Build history of the part. All positions in model axes, mm. A direction names the side the tool comes from. Round coordinates to 2 decimals unless told otherwise and drop trailing zeros. Loops run counter-clockwise (first coordinate to the right, second up) from the corner with the lowest first, then second, coordinate; pieces in that order, holes last.
from build123d import *

# Parameters (mm, degrees)
CROQUIS1_R              = 44.1
CROQUIS1_R_2            = 15.875
SALIENTE_EXTRUIR1_DEPTH = 15.875
SALIENTE_EXTRUIR2_DEPTH = 15.875
MATRIZC1_DEPTH          = 15.875


# Read off the part's stored shape, not the designer's step: MatrizC1
with BuildPart() as part:
    # Croquis1 → Saliente-Extruir1 (new body)
    with BuildSketch(Plane.XY):
        Circle(CROQUIS1_R)
        Circle(CROQUIS1_R_2, mode=Mode.SUBTRACT)
    extrude(amount=SALIENTE_EXTRUIR1_DEPTH)

    # Croquis2 → Saliente-Extruir2 (add)
    with BuildSketch(Plane.XY.offset(15.875)):
        Polygon((-1, 50.6), (1, 50.6), (2.815859205, 42.731276779), (-2.815859205, 42.731276779), align=None)
    extrude(amount=-SALIENTE_EXTRUIR2_DEPTH)

    # MatrizC1 outline → MatrizC1 (add)
    with BuildSketch(Plane.XY):
        with BuildLine():
            ThreePointArc((-13.826153616, 41.876574313), (-11.413919889, 42.59732894), (-8.964486889, 43.179253987))
            Line((-8.964486889, 43.179253987), (-12.130317856, 49.134665855))
            Line((-12.130317856, 49.134665855), (-14.062169508, 48.617027765))
            Line((-14.062169508, 48.617027765), (-13.826153616, 41.876574313))
        make_face()
        with BuildLine():
            ThreePointArc((8.964486889, 43.179253987), (11.413919889, 42.59732894), (13.826153616, 41.876574313))
            Line((13.826153616, 41.876574313), (14.062169508, 48.617027765))
            Line((14.062169508, 48.617027765), (12.130317856, 49.134665855))
            Line((12.130317856, 49.134665855), (8.964486889, 43.179253987))
        make_face()
        with BuildLine():
            ThreePointArc((19.83464269, 39.387776649), (22.05, 38.191720307), (24.193493831, 36.87119277))
            Line((24.193493831, 36.87119277), (26.166025404, 43.320885431))
            Line((26.166025404, 43.320885431), (24.433974596, 44.320885431))
            Line((24.433974596, 44.320885431), (19.83464269, 39.387776649))
        make_face()
        with BuildLine():
            ThreePointArc((29.353100371, 32.912087424), (31.18340905, 31.18340905), (32.912087424, 29.353100371))
            Line((32.912087424, 29.353100371), (36.486709909, 35.072496347))
            Line((36.486709909, 35.072496347), (35.072496347, 36.486709909))
            Line((35.072496347, 36.486709909), (29.353100371, 32.912087424))
        make_face()
        with BuildLine():
            ThreePointArc((36.87119277, 24.193493831), (38.191720307, 22.05), (39.387776649, 19.83464269))
            Line((39.387776649, 19.83464269), (44.320885431, 24.433974596))
            Line((44.320885431, 24.433974596), (43.320885431, 26.166025404))
            Line((43.320885431, 26.166025404), (36.87119277, 24.193493831))
        make_face()
        with BuildLine():
            ThreePointArc((41.876574313, 13.826153616), (42.597328939, 11.413919889), (43.179253986, 8.964486889))
            Line((43.179253986, 8.964486889), (49.134665855, 12.130317856))
            Line((49.134665855, 12.130317856), (48.617027765, 14.062169508))
            Line((48.617027765, 14.062169508), (41.876574313, 13.826153616))
        make_face()
        with BuildLine():
            ThreePointArc((44.028136522, 2.51658388), (44.1, 0), (44.028136522, -2.51658388))
            Line((44.028136522, -2.51658388), (50.6, -1))
            Line((50.6, -1), (50.6, 1))
            Line((50.6, 1), (44.028136522, 2.51658388))
        make_face()
        with BuildLine():
            ThreePointArc((43.179253986, -8.964486889), (42.597328939, -11.413919889), (41.876574313, -13.826153616))
            Line((41.876574313, -13.826153616), (48.617027765, -14.062169508))
            Line((48.617027765, -14.062169508), (49.134665855, -12.130317856))
            Line((49.134665855, -12.130317856), (43.179253986, -8.964486889))
        make_face()
        with BuildLine():
            ThreePointArc((39.387776649, -19.83464269), (38.191720307, -22.05), (36.871192769, -24.193493831))
            Line((36.871192769, -24.193493831), (43.320885431, -26.166025404))
            Line((43.320885431, -26.166025404), (44.320885431, -24.433974596))
            Line((44.320885431, -24.433974596), (39.387776649, -19.83464269))
        make_face()
        with BuildLine():
            ThreePointArc((32.912087424, -29.353100371), (31.18340905, -31.18340905), (29.353100371, -32.912087424))
            Line((29.353100371, -32.912087424), (35.072496347, -36.486709909))
            Line((35.072496347, -36.486709909), (36.486709909, -35.072496347))
            Line((36.486709909, -35.072496347), (32.912087424, -29.353100371))
        make_face()
        with BuildLine():
            ThreePointArc((24.193493831, -36.871192769), (22.05, -38.191720307), (19.83464269, -39.387776649))
            Line((19.83464269, -39.387776649), (24.433974596, -44.320885431))
            Line((24.433974596, -44.320885431), (26.166025404, -43.320885431))
            Line((26.166025404, -43.320885431), (24.193493831, -36.871192769))
        make_face()
        with BuildLine():
            ThreePointArc((13.826153616, -41.876574313), (11.413919889, -42.597328939), (8.964486889, -43.179253986))
            Line((8.964486889, -43.179253986), (12.130317856, -49.134665855))
            Line((12.130317856, -49.134665855), (14.062169508, -48.617027765))
            Line((14.062169508, -48.617027765), (13.826153616, -41.876574313))
        make_face()
        with BuildLine():
            ThreePointArc((2.51658388, -44.028136522), (0, -44.1), (-2.51658388, -44.028136522))
            Line((-2.51658388, -44.028136522), (-1, -50.6))
            Line((-1, -50.6), (1, -50.6))
            Line((1, -50.6), (2.51658388, -44.028136522))
        make_face()
        with BuildLine():
            ThreePointArc((-8.964486889, -43.179253986), (-11.413919889, -42.597328939), (-13.826153616, -41.876574313))
            Line((-13.826153616, -41.876574313), (-14.062169508, -48.617027765))
            Line((-14.062169508, -48.617027765), (-12.130317856, -49.134665855))
            Line((-12.130317856, -49.134665855), (-8.964486889, -43.179253986))
        make_face()
        with BuildLine():
            ThreePointArc((-19.83464269, -39.387776649), (-22.05, -38.191720307), (-24.193493831, -36.871192769))
            Line((-24.193493831, -36.871192769), (-26.166025404, -43.320885431))
            Line((-26.166025404, -43.320885431), (-24.433974596, -44.320885431))
            Line((-24.433974596, -44.320885431), (-19.83464269, -39.387776649))
        make_face()
        with BuildLine():
            ThreePointArc((-29.353100371, -32.912087424), (-31.18340905, -31.18340905), (-32.912087424, -29.353100371))
            Line((-32.912087424, -29.353100371), (-36.486709909, -35.072496347))
            Line((-36.486709909, -35.072496347), (-35.072496347, -36.486709909))
            Line((-35.072496347, -36.486709909), (-29.353100371, -32.912087424))
        make_face()
        with BuildLine():
            ThreePointArc((-36.871192769, -24.193493831), (-38.191720307, -22.05), (-39.387776649, -19.83464269))
            Line((-39.387776649, -19.83464269), (-44.320885431, -24.433974596))
            Line((-44.320885431, -24.433974596), (-43.320885431, -26.166025404))
            Line((-43.320885431, -26.166025404), (-36.871192769, -24.193493831))
        make_face()
        with BuildLine():
            ThreePointArc((-41.876574313, -13.826153616), (-42.597328939, -11.413919889), (-43.179253986, -8.964486889))
            Line((-43.179253986, -8.964486889), (-49.134665855, -12.130317856))
            Line((-49.134665855, -12.130317856), (-48.617027765, -14.062169508))
            Line((-48.617027765, -14.062169508), (-41.876574313, -13.826153616))
        make_face()
        with BuildLine():
            ThreePointArc((-44.028136522, -2.51658388), (-44.1, 0), (-44.028136522, 2.51658388))
            Line((-44.028136522, 2.51658388), (-50.6, 1))
            Line((-50.6, 1), (-50.6, -1))
            Line((-50.6, -1), (-44.028136522, -2.51658388))
        make_face()
        with BuildLine():
            ThreePointArc((-43.179253986, 8.964486889), (-42.597328939, 11.413919889), (-41.876574313, 13.826153616))
            Line((-41.876574313, 13.826153616), (-48.617027765, 14.062169508))
            Line((-48.617027765, 14.062169508), (-49.134665855, 12.130317856))
            Line((-49.134665855, 12.130317856), (-43.179253986, 8.964486889))
        make_face()
        with BuildLine():
            ThreePointArc((-39.387776649, 19.83464269), (-38.191720307, 22.05), (-36.87119277, 24.193493831))
            Line((-36.87119277, 24.193493831), (-43.320885431, 26.166025404))
            Line((-43.320885431, 26.166025404), (-44.320885431, 24.433974596))
            Line((-44.320885431, 24.433974596), (-39.387776649, 19.83464269))
        make_face()
        with BuildLine():
            ThreePointArc((-32.912087424, 29.353100371), (-31.18340905, 31.18340905), (-29.353100371, 32.912087424))
            Line((-29.353100371, 32.912087424), (-35.072496347, 36.486709909))
            Line((-35.072496347, 36.486709909), (-36.486709909, 35.072496347))
            Line((-36.486709909, 35.072496347), (-32.912087424, 29.353100371))
        make_face()
        with BuildLine():
            ThreePointArc((-24.193493831, 36.87119277), (-22.05, 38.191720307), (-19.83464269, 39.387776649))
            Line((-19.83464269, 39.387776649), (-24.433974596, 44.320885431))
            Line((-24.433974596, 44.320885431), (-26.166025404, 43.320885431))
            Line((-26.166025404, 43.320885431), (-24.193493831, 36.87119277))
        make_face()
    extrude(amount=MATRIZC1_DEPTH)


solid = part.part
(1) Probe line 1 (X direction, y = 33.5, z = 1.5); line 2 (Y direction, x = 0, z = 8) (3 decimals); line 3 (Y direction, x = -43, z = 7.75). List the from-to ranges inside material, lowest first.
Responses:
line 1: x = -35.5 to -30.29, -28.68 to 28.68, 30.29 to 35.5
line 2: y = -50.6 to -15.875, 15.875 to 50.6
line 3: y = -26.07 to -23.2, -13.87 to 13.87, 23.2 to 26.07
(2) Pull direction X, two halves, no side cores. Call faces 1 (the face through (-43.73, -5.71, 7.83)), 2 (the face through (-35.015, -26.81, 7.826)), 3 (the face through (25.166, 40.051, 7.826)): +X half, -X half, draft (parallel to the pull), parting line (faces both ways), or undercut.
Responses:
face 1: -X half
face 2: undercut
face 3: +X half
(3) Slice it at B-B on x = 22. List the corners of the cut face in (y, z) (3 decimals), plus the area to 3 significant figures.
Responses:
outline: (-41.71, 0) - (41.71, 0) - (41.71, 15.875) - (-41.71, 15.875) - close
area: 1,320 mm2
(4) Which spindle directions (+Z, -Z, +X, -X, +Y, -Y) get a long thin tool onto all of the face, cutting with end or side? Do faces 4 (the face through (47.27, -1.77, 7.83)), 5 (the face through (34.96, -26.88, 7.83)), 6 (the face through (1.748, -47.36, 7.826)), 7 (the face through (-43.717, 5.801, 7.826)), 8 (the face through (1.748, 47.36, 8.049)). Say none if no direction does.
Responses:
face 4: +Z, -Z, +X
face 5: +Z, -Z
face 6: +Z, -Z, -Y
face 7: +Z, -Z, -X
face 8: +Z, -Z, +Y
(5) Slice it at A-A on x = -4.5. List the corners of the cut face in (y, z) (3 decimals), plus the area to 3 significant figures.
Responses:
outline: (-43.87, 0) - (-15.224, 0) - (-15.224, 15.875) - (-43.87, 15.875) - close; (15.224, 0) - (43.87, 0) - (43.87, 15.875) - (15.224, 15.875) - close
area: 910 mm2
(6) Pin check, flat tips, straight feed: P1, Ø1.5, axis at x = 21, z = 14, coming from the +Y side; P2, Ø5, axis at y = 13.5, z = 3, coming from the -X side; P3, Ø3, axis at x = -16, z = 9.5, coming from the +Y side. Stop position of each tip, or through.
Responses:
P1: stops at y = 41.44
P2: stops at x = -49.13
P3: stops at y = 41.65
